from build123d import *

# Parameters (mm, degrees)
F0_R     = 19.84375
F1_DEPTH = 6.35
F2_T     = -1.5875
F4_DEPTH = 7.9375
F6_R     = 19.84375
F7_DEPTH = 6.35


with BuildPart() as f1:
    # F0 (on Top) → F1 (new body)
    with BuildSketch(Plane.XY):
        Circle(F0_R)
    extrude(amount=F1_DEPTH)

    # F2
    f2_openings = [f1.faces().sort_by_distance(p)[0] for p in [
        (0, 0, 6.35),
    ]]
    offset(amount=F2_T, openings=f2_openings)

    # F3 (on face) → F4 (join)
    with BuildSketch(Plane.XY.offset(1.5875)):
        with BuildLine():
            Line((2.776140625, -5.55625), (2.776140625, 5.55625))
            ThreePointArc((2.776140625, 5.55625), (-3.573859375, 0), (2.776140625, -5.55625))
        make_face()
        with BuildLine():
            Line((2.032, 3.429), (2.032, -3.429))
            ThreePointArc((2.032, -3.429), (-2.032, 0), (2.032, 3.429))
        make_face(mode=Mode.SUBTRACT)
    extrude(amount=F4_DEPTH)

    # F6 (on face) → F7 (join)
    with BuildSketch(Plane(origin=(0, 0, 0), x_dir=(1, 0, 0), z_dir=(0, 0, -1))):
        Circle(F6_R)
    extrude(amount=F7_DEPTH)


solid = f1.part
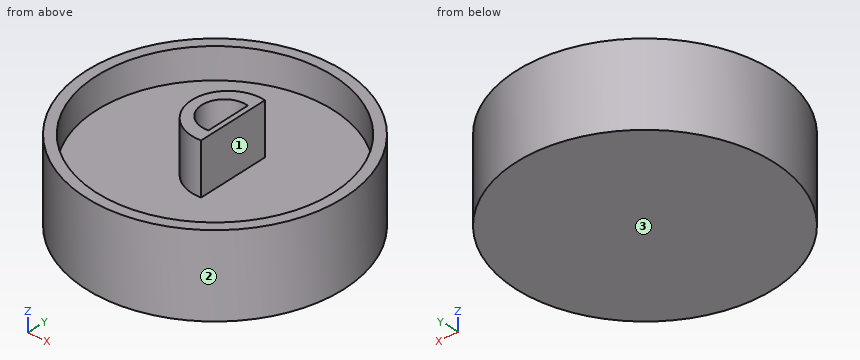
Design review of the part built by this model. Coordinates are the model's own, in mm. Face numbers are marked on the shaded views. Coordinates: 2 decimals unless noted, no trailing zeros. Loops run counter-clockwise (first coordinate to the right, second up) from the corner with the lowest first, then second, coordinate; pieces in that order, holes last.
Item 1: Add section C-C (z = 7). Write out the cut boundary in (x, y).
Completed:
outline: (2.78, -5.56) - (2.78, 5.56) arc R5.61 ccw (long way) to start; hole (2.03, -3.43) - (2.03, 3.43) arc R3.48 ccw (long way) to start
Item 2: Clearance check with flat-ended pins moving along their axes: pin 1 (1 mm diameter, centred on y = 7.5, z = 6, fed in from +X); pin 2 (4 mm diameter, centred on x = -3, z = -3.5, fed in from -Y); pin 3 (10 mm diameter, centred on x = -7, y = -15, fed in from +Z); pin 4 (5.5 mm diameter, centred on y = 0.5, z = 6, fed in from -X). State where each tip first meets the part, or that it passes through.
Completed:
pin 1: stops at x = 18.57
pin 2: stops at y = -19.82
pin 3: stops at z = 6.35
pin 4: stops at x = -19.84
Item 3: Add section D-D (z = 1). Write out the cut boundary in (x, y), and give its area (3 significant figures).
Completed:
outline: circle Ø39.69 at (0, 0)
area: 1,240 mm2
Item 4: Add section B-B (x = -9). Write out the cut boundary in (y, z).
Completed:
outline: (-17.69, -6.35) - (17.69, -6.35) - (17.69, 6.35) - (15.88, 6.35) - (15.88, 1.59) - (-15.88, 1.59) - (-15.88, 6.35) - (-17.69, 6.35) - close
Item 5: Draft analysis for pull direction Y (two halves, no side actions). For the marked faces 1, 2 and 3, state which applies: pulls with the +Y half, pulls with the -Y half, needs draft (parallel to the pull), parting line crosses it, or undercut.
Completed:
face 1: undercut
face 2: parting line crosses it
face 3: needs draft
Item 6: Wall thickness on L1, parallel to X at y = 0, z = 3.25; L2, parallel to Y at x = 0, z = 3.5; L3, parallel to Y at x = -3, z = 5.5: over which ranges is each line inside the solid? List them lowest first.
Completed:
L1: x = -19.84 to -18.26, -3.57 to -2.03, 2.03 to 2.78, 18.26 to 19.84
L2: y = -19.84 to -18.26, -5.22 to -3.16, 3.16 to 5.22, 18.26 to 19.84
L3: y = -19.62 to -18.01, -2.47 to 2.47, 18.01 to 19.62
